Geometry: see drawing. Coordinates: mm, zero at the bounding-box minimum. A direction names the side the tool comes from. Round coordinates to 2 decimals unless told otherwise and drop trailing zeros. Write each loop counter-clockwise with the first axis right and the second up, starting at its lowest first coordinate (ties: lowest second). Pieces come first, ordered by that corner, then holes.
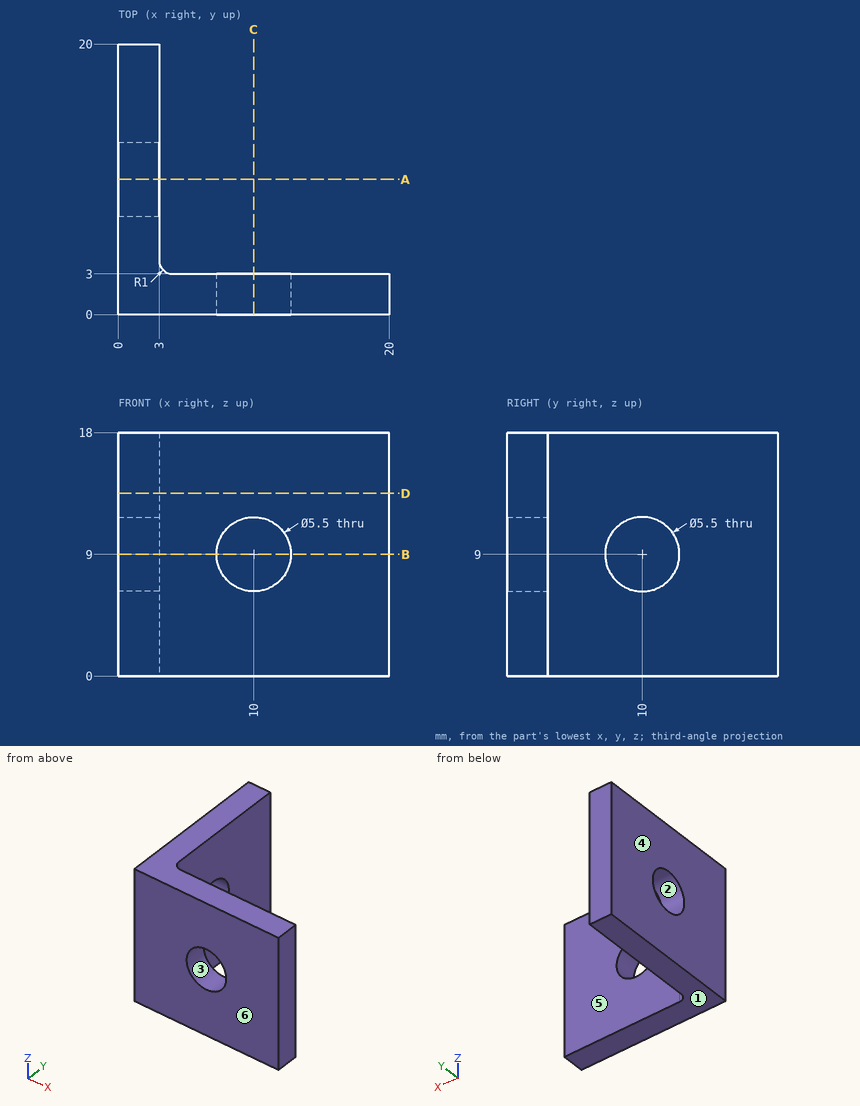
1) Section query B-B on z = 9. Return the cut outline in (x, y), then the cut area to 3 significant figures.
Taken from the geometry:
outline: (0, 0) - (7.25, 0) - (7.25, 3) - (4, 3) arc R1 cw to (3, 4) - (3, 7.25) - (0, 7.25) - close; (0, 12.75) - (3, 12.75) - (3, 20) - (0, 20) - close; (12.75, 0) - (20, 0) - (20, 3) - (12.75, 3) - close
area: 78.2 mm2
2) Material intervals for line 1 (X direction, y = 2.05, z = 9); line 2 (Z direction, x = 10, y = 1.1), sorted ascending.
Taken from the geometry:
line 1: x = 0 to 7.25, 12.75 to 20
line 2: z = 0 to 6.25, 11.75 to 18
3) Reachability of the marked faces 5 and 6 from +Z, -Z, +X, -X, +Y, -Y: full face, straight path, thin tool, end or side. Return the list, or none.
Taken from the geometry:
face 5: +Z, -Z, +X, +Y
face 6: +Z, -Z, +X, -X, -Y
4) Contact query for flat-ended pins moving along their axis: P1, Ø1.5, axis at y = 10.5, z = 13, coming from the +X side; P2, Ø5, axis at y = 10, z = 9, coming from the +X side. Output: stop coordinate, or through.
Taken from the geometry:
P1: stops at x = 3
P2: passes through
5) Section query A-A on y = 10. Return the cut outline in (x, z).
Taken from the geometry:
outline: (0, 0) - (3, 0) - (3, 6.25) - (0, 6.25) - close; (0, 11.75) - (3, 11.75) - (3, 18) - (0, 18) - close
6) Section query D-D on z = 13.5. Return the cut outline in (x, y), then the cut area to 3 significant figures.
Taken from the geometry:
outline: (0, 0) - (20, 0) - (20, 3) - (4, 3) arc R1 cw to (3, 4) - (3, 20) - (0, 20) - close
area: 111 mm2
7) Pull-direction query (Z, two-part tool) for the marked faces 1, 2, 3 and 4; classes: released by +Z, released by -Z, zero draft, split by the parting line, or undercut.
Taken from the geometry:
face 1: released by -Z
face 2: undercut
face 3: undercut
face 4: zero draft
